The model under review builds one solid part; all positions refer to its coordinate system, in mm. Face numbers are marked on the shaded views. A direction names the side the tool comes from. Coordinates: 2 decimals unless noted, no trailing zeros. Loops run counter-clockwise (first coordinate to the right, second up) from the corner with the lowest first, then second, coordinate; pieces in that order, holes last. Notation, with made-up numbers: (-33.75, -37) - (-14.75, -37) arc R17 ccw to (-14.75, -14) - close; hole circle Ø3 at (55, -37). An arc over 180 degrees is marked (long way). Use a Markdown table: item, result. Add a question column.
1) Clearance check with flat-ended pins moving along their axes: pin 1 (1.5 mm diameter, centred on y = -1, z = -1.5, fed in from +X); pin 2 (2 mm diameter, centred on x = -3, z = -3.5, fed in from +Y). State where each tip first meets the part, or that it passes through.
2) For the marked faces 4 and 5, list the 3-axis set-ups (+Z, -Z, +X, -X, +Y, -Y) from which the entire face can be reached by the end or side of a thin tool; tool diameter is ignored.
3) The part is to be moulded in two halves that separate along Y. For the marked faces 1, 2 and 3, say which applies: pulls with the +Y half, pulls with the -Y half, needs draft (parallel to the pull), parting line crosses it, or undercut.
4) Add section C-C, the plane z = -1.75. Give the boundary of the cut face in (x, y), and give its area (3 significant figures).
5) Add section A-A, the plane x = 0. Give the boundary of the cut face in (y, z), and give its area (3 significant figures).
6) Add section D-D, the plane x = 7.5. Give the boundary of the cut face in (y, z).
7) To check wall thickness, follow L1, parallel to Z at x = 0.25, y = 7; L2, parallel to Y at x = 0, z = 0.5; L3, parallel to X at y = 1.75, z = -1.25. State the ranges of each line that lie inside material, in increasing order. Write a range as [from, to].
```python
from build123d import *

# Parameters (mm, degrees)
CYLINDER003_R     = 2.5
CYLINDER003_DEPTH = 10
CYLINDER001_R     = 9
CYLINDER001_DEPTH = 1
CYLINDER_R        = 6
CYLINDER_DEPTH    = 6.4
CYLINDER002_R     = 9
CYLINDER002_DEPTH = 1


with BuildPart() as cilindro003:
    # Cylinder003 → Cylinder003 (new body)
    with BuildSketch(Plane.XY.offset(-5)):
        Circle(CYLINDER003_R)
    extrude(amount=CYLINDER003_DEPTH)


with BuildPart() as cilindro001:
    # Cylinder001 → Cylinder001 (new body)
    with BuildSketch(Plane.XY.offset(3.2)):
        Circle(CYLINDER001_R)
    extrude(amount=CYLINDER001_DEPTH)


with BuildPart() as fusion:
    # Cylinder → Cylinder (new body)
    with BuildSketch(Plane.XY.offset(-3.2)):
        Circle(CYLINDER_R)
    extrude(amount=CYLINDER_DEPTH)

    # Fusion: union Cilindro001
    add(cilindro001.part)


with BuildPart() as pulley:
    # Cylinder002 → Cylinder002 (new body)
    with BuildSketch(Plane.XY.offset(-4.2)):
        Circle(CYLINDER002_R)
    extrude(amount=CYLINDER002_DEPTH)

    # Fusion001: union Fusion
    add(fusion.part)

    # Cut: cut Cilindro003
    add(cilindro003.part, mode=Mode.SUBTRACT)


solid = pulley.part
```
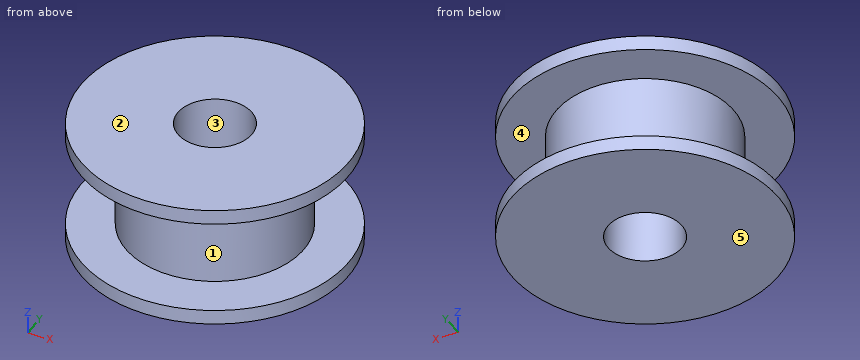
From the geometry:
| question | item | result |
|---|---|---|
| 1 | pin 1 | stops at x = 5.99 |
| 1 | pin 2 | stops at y = 8.77 |
| 2 | face 4 | none |
| 2 | face 5 | -Z, +X, -X, +Y, -Y |
| 3 | face 1 | parting line crosses it |
| 3 | face 2 | needs draft |
| 3 | face 3 | undercut |
| 4 | outline | circle Ø12 at (0, 0); hole circle Ø5 at (0, 0) |
| 4 | area | 93.5 mm^2 |
| 5 | outline | (-9, -4.2) - (-2.5, -4.2) - (-2.5, 4.2) - (-9, 4.2) - (-9, 3.2) - (-6, 3.2) - (-6, -3.2) - (-9, -3.2) - close; (2.5, -4.2) - (9, -4.2) - (9, -3.2) - (6, -3.2) - (6, 3.2) - (9, 3.2) - (9, 4.2) - (2.5, 4.2) - close |
| 5 | area | 70.8 mm^2 |
| 6 | outline | (-4.97, -4.2) - (4.97, -4.2) - (4.97, -3.2) - (-4.97, -3.2) - close; (-4.97, 3.2) - (4.97, 3.2) - (4.97, 4.2) - (-4.97, 4.2) - close |
| 7 | L1 | z = [-4.2, -3.2], [3.2, 4.2] |
| 7 | L2 | y = [-6, -2.5], [2.5, 6] |
| 7 | L3 | x = [-5.74, -1.79], [1.79, 5.74] |
